Autodesk Inventor part; units mm, degrees
ref_plane "YZ Plane" through (0, 0, 0) normal (1, 0, 0) x (0, 1, 0)
ref_plane "XZ Plane" through (0, 0, 0) normal (0, 1, 0) x (-1, 0, 0)
ref_plane "XY Plane" through (0, 0, 0) normal (0, 0, 1) x (1, 0, 0)
sketch "Sketch_1" plane through (0, 0, 0) normal (0, 0, 1) x (1, 0, 0)
  line L0 (100, 0) -> (0, 0)
  line L1 (0, 4.5) -> (0, 2)
  line L2 (0, 2) -> (100, 2)
  line L3 (100, 2) -> (100, 4.5)
  line L4 (100, 4.5) -> (99.5, 5)
  line L5 (99.5, 5) -> (0.5, 5)
  line L6 (0.5, 5) -> (0, 4.5)
revolve "Revolution1" add sketch "Sketch_1" angle 360 about axis through (100, 0, 0) along (1, 0, 0)
sketch "Sketch_6" plane through (0, 0, 0) normal (0, 0, 1) x (1, 0, 0)
  line L0 (12.5, 0) -> (0, 0)
  line L1 (0, 0) -> (0, 2.5)
  line L2 (0, 2.5) -> (0.433, 2.067)
  line L3 (0.433, 2.067) -> (11.3066, 2.067)
  line L4 (11.3066, 2.067) -> (12.5, 0)
  line L5 (12.5, 0) -> (0, 0)
revolve "Revolution2" cut sketch "Sketch_6" angle 360 about axis through (12.5, 0, 0) along (1, 0, 0)
thread "Thread1"
sketch "Sketch_7" plane through (0, 0, 0) normal (0, 0, 1) x (1, 0, 0)
  line L0 (100, 0) -> (85, 0)
  line L1 (85, 0) -> (86.4194, 2.4585)
  line L2 (86.4194, 2.4585) -> (99.4585, 2.4585)
  line L3 (99.4585, 2.4585) -> (100, 3)
  line L4 (100, 3) -> (100, 0)
  line L5 (100, 0) -> (85, 0)
revolve "Revolution3" cut sketch "Sketch_7" angle 360 about axis through (100, 0, 0) along (1, 0, 0)
thread "Thread2"
sketch "Sketch_2" plane through (10, 0, 0) normal (1, 0, 0) x (0, 0, -1)
  line L0 (-6, 7) -> (-6, -5)
  line L1 (-6, -5) -> (-4, -5)
  line L2 (-4, -5) -> (-4, 6)
  line L3 (-4, 6) -> (4, 6)
  line L4 (4, 6) -> (4, -5)
  line L5 (4, -5) -> (6, -5)
  line L6 (6, -5) -> (6, 7)
  line L7 (6, 7) -> (-6, 7)
extrude "Extrusion1" cut sketch "Sketch_2" along normal blind 8
properties part number "PSPWR10-100-M5-N6-SC10" material "MISUMI"
Verification items for the finished model (mm, model axes). A direction names the side the tool comes from. Give positions to 0.01 mm unless a question says otherwise; leave off trailing zeros. Write each loop counter-clockwise with the first axis right and the second up, starting at its lowest first coordinate (ties: lowest second). Pieces come first, ordered by that corner, then holes. Notation, with made-up numbers: M 41.5,53.25 L 92.5,53.25 A9 ccw 92.5,63.25 Z; hole C -38.75,-5 d5. An arc over 180 degrees is marked long. One line per question, with ' | ' between items.
1) Gauge pin test, flat ends, axial feed: pin 1 Ø3.5 at (y, z) = (0, 0) entering from +X; pin 2 Ø2 at (x, y) = (71, -4) entering from +Z; pin 3 Ø1.8 at (x, y) = (13, -1) entering from -Z; pin 4 Ø1 at (x, z) = (37, 2) entering from -Y. Record the tip position at first contact, or that the pin passes through.
Result:
pin 1: passes through | pin 2: stops at z = 4 | pin 3: stops at z = -4 | pin 4: stops at y = -4.77
2) Set-up check for faces 1 (the flat face through (100, 1, -3)), 2 (the cylindrical face through (93.03, 2.345, 0.738)), 3 (the flat face through (14, 0, -4)): record each of +Z, -Z, +X, -X, +Y, -Y from which the full face is reachable in a straight line by a thin tool's end or side.
Result:
face 1: +Z, -Z, +X, +Y, -Y | face 2: +X | face 3: -Z, +Y, -Y
3) Section check D-D on x = 79. Enter the section's corners in (y, z).
Result:
outline: C 0,0 d10; hole C 0,0 d4
4) Section check B-B on z = 0. Enter the section's corners in (x, y), plus the area to 3 significant figures.
Result:
outline: M 0,-4.5 L 0.5,-5 L 99.5,-5 L 100,-4.5 L 100,-3 L 99.46,-2.46 L 86.42,-2.46 L 86.15,-2 L 11.35,-2 L 11.31,-2.07 L 0.43,-2.07 L 0,-2.5 Z; M 0,2.5 L 0.43,2.07 L 11.31,2.07 L 11.35,2 L 86.15,2 L 86.42,2.46 L 99.46,2.46 L 100,3 L 100,4.5 L 99.5,5 L 0.5,5 L 0,4.5 Z | area: 585 mm2
5) Mould release check, pull along Y, two halves, no side actions. Record for faces 4 (the flat face through (14, 0, 4)), 5 (the cylindrical face through (5.95, -1.64, -1.26)), 6 (the cylindrical face through (49, -5, 0)): released by +Y, released by -Y, zero draft, split by the parting line, or undercut.
Result:
face 4: zero draft | face 5: undercut | face 6: split by the parting line
6) Thickness scan on line 1 along Z through (x, y) = (5, 0); line 2 along Z through (x, y) = (46, 3); line 3 along Y through (x, z) = (41.5, 0.25). Record the ranges inside material, lowest first. Write a range as [from, to].
Result:
line 1: z = [-5, -2.07], [2.07, 5] | line 2: z = [-4, 4] | line 3: y = [-4.99, -1.98], [1.98, 4.99]
7) Section check C-C on x = 14.5. Enter the section's corners in (y, z), plus the area to 3 significant figures.
Result:
outline: M -3,-4 L 3,-4 A5 ccw 3,4 L -3,4 A5 ccw Z; hole C 0,0 d4 | area: 57.8 mm2
